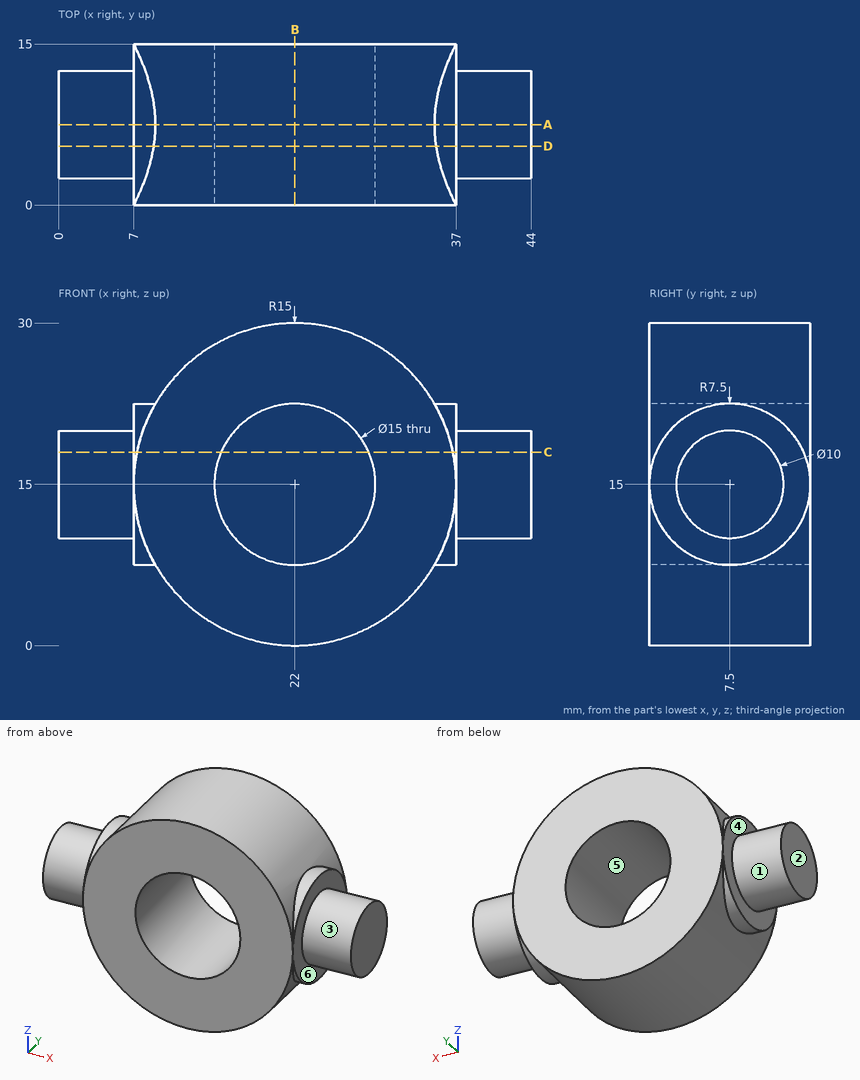
Job drawing, mm, ordinate dimensions from the low corner. One solid piece. A direction names the side the tool comes from. Round coordinates to 2 decimals unless told otherwise and drop trailing zeros. Loops run counter-clockwise (first coordinate to the right, second up) from the corner with the lowest first, then second, coordinate; pieces in that order, holes last.
Item 1: Cut at C-C, the plane z = 18. Give the cut face in (x, y).
Item 2: Drill centre lines: line 1 (Z direction, x = 22, y = 11); line 2 (X direction, y = 6, z = 10.5); line 3 (Z direction, x = 16, y = 4). Where is each one in solid material? Low to high.
Item 3: Mould opens along X. For the marked faces 4, 5 and 6 say: +X half, -X half, draft (parallel to the pull), parting line (faces both ways), or undercut.
Item 4: Cut at A-A, the plane y = 7.5. Give the cut face in (x, z).
Item 5: 3-axis set-ups, long thin cutter, end or side, ignore diameter. For the marked faces 1, 2 and 3: which of +Z, -Z, +X, -X, +Y, -Y reach the whole face in a straight line?
Item 6: Cut at B-B, the plane x = 22. Give the cut face in (y, z).
Item 7: Drop flat-ended pins along their axis: P1, Ø4, axis at x = 14, y = 9.5, coming from the +Z side; P2, Ø12, axis at x = 22, z = 15, coming from the -Y side; P3, Ø6, axis at x = 12, y = 12.5, coming from the +Z side; P4, Ø1, axis at y = 9, z = 8.5, coming from the -X side. Give the stop position or say it passes through.
Item 8: Cut at D-D, the plane y = 5.5. Give the cut face in (x, z).
A:
1. outline: (0, 3.5) - (7, 3.5) - (7, 0.63) - (7.3, 0.63) - (7.3, 0) - (15.13, 0) - (15.13, 15) - (7.3, 15) - (7.3, 14.37) - (7, 14.37) - (7, 11.5) - (0, 11.5) - close; (28.87, 0) - (36.7, 0) - (36.7, 0.63) - (37, 0.63) - (37, 3.5) - (44, 3.5) - (44, 11.5) - (37, 11.5) - (37, 14.37) - (36.7, 14.37) - (36.7, 15) - (28.87, 15) - close
2. line 1: z = 0 to 7.5, 22.5 to 30
2. line 2: x = 0 to 16, 28 to 44
2. line 3: z = 1.25 to 10.5, 19.5 to 28.75
3. face 4: -X half
3. face 5: undercut
3. face 6: +X half
4. outline: (0, 10) - (7, 10) - (7, 7.5) - (9.01, 7.5) arc R15 ccw to (34.99, 7.5) - (37, 7.5) - (37, 10) - (44, 10) - (44, 20) - (37, 20) - (37, 22.5) - (34.99, 22.5) arc R15 ccw to (9.01, 22.5) - (7, 22.5) - (7, 20) - (0, 20) - close; hole circle Ø15 at (22, 15)
5. face 1: -X
5. face 2: +Z, -Z, -X, +Y, -Y
5. face 3: +X
6. outline: (0, 0) - (15, 0) - (15, 7.5) - (0, 7.5) - close; (0, 22.5) - (15, 22.5) - (15, 30) - (0, 30) - close
7. P1: stops at z = 28.75
7. P2: passes through
7. P3: stops at z = 28.27
7. P4: stops at x = 7
8. outline: (0, 10.42) - (7, 10.42) - (7, 7.77) - (8.86, 7.77) arc R15 ccw to (35.14, 7.77) - (37, 7.77) - (37, 10.42) - (44, 10.42) - (44, 19.58) - (37, 19.58) - (37, 22.23) - (35.14, 22.23) arc R15 ccw to (8.86, 22.23) - (7, 22.23) - (7, 19.58) - (0, 19.58) - close; hole circle Ø15 at (22, 15)
